Check sheet for the drawn part. Datum: minimum x, y, z corner. Units: mm. Coordinates: 2 decimals unless noted, no trailing zeros. Order: outer loops, then holes, each group sorted by start corner. A loop starts at its lowest first (then second) coordinate and runs counter-clockwise, first axis right, second up. Notation, with made-up numbers: M 28,-10 L 42,-10 A25 ccw 42,9 Z; hole C 60.25,20 d4. An arc over 180 degrees is marked long. Answer in a Markdown table with one row per item. Add a question column.
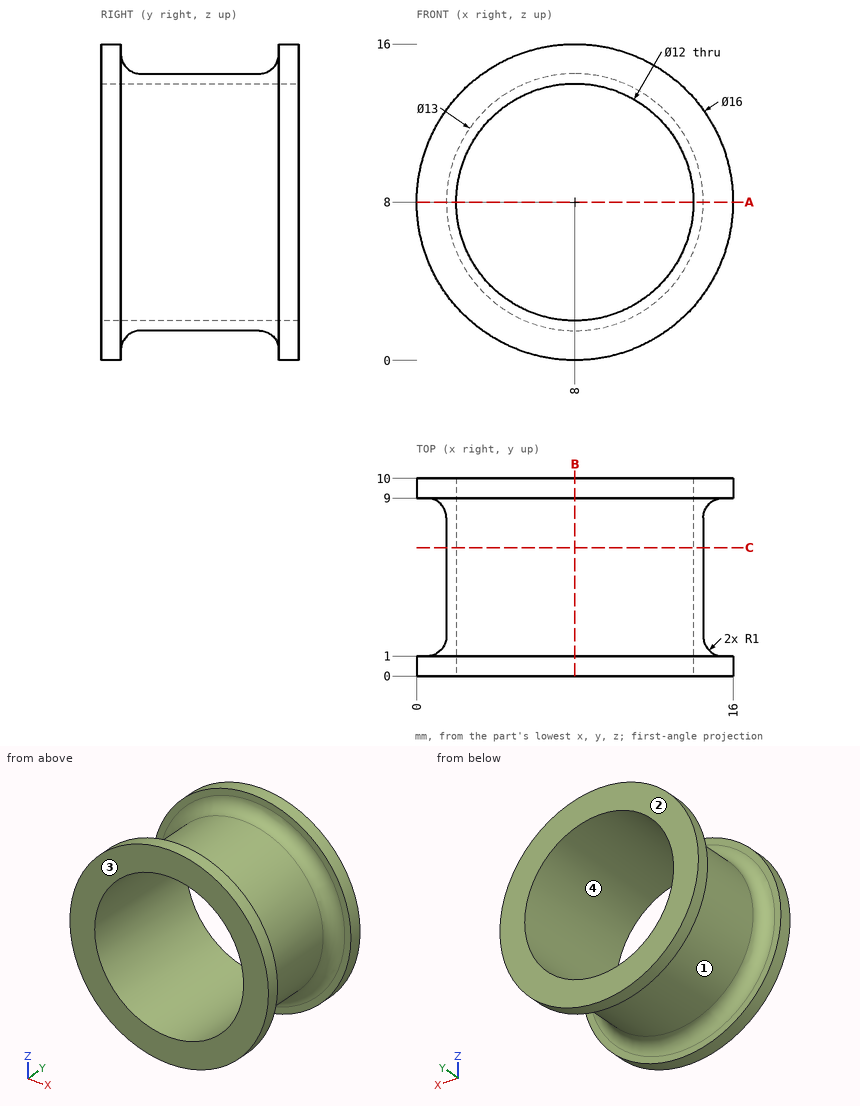
1. Section check C-C on y = 6.5. Enter the section's corners in (x, z), then the cut area to 3 significant figures.
2. Section check B-B on x = 8. Enter the section's corners in (y, z).
3. Release check for a two-part mould opening along Y. For the marked faces 1, 2, 3 and 4 record: released by +Y, released by -Y, zero draft, split by the parting line, or undercut.
4. Scan lines: line 1 (X direction, y = 2.75, z = 8); line 2 (Y direction, x = 12.75, z = 14.25); line 3 (Y direction, x = 1.75, z = 4.75). Record each from-to range of solid material in increasing order.
5. Section check A-A on z = 8. Enter the section's corners in (x, y).
6. Go/stop test with flat-tipped pins: pin 1 Ø1 at (y, z) = (2, 5) entering from +X; pin 2 Ø6 at (x, y) = (4.5, 7) entering from -Z. Record where each tip stops, or that it passes through.
Result sheet:
| question | item | result |
|---|---|---|
| 1 | outline | C 8,8 d13; hole C 8,8 d12 |
| 1 | area | 19.6 mm^2 |
| 2 | outline | M 0,0 L 1,0 L 1,0.5 A1 cw 2,1.5 L 8,1.5 A1 cw 9,0.5 L 9,0 L 10,0 L 10,2 L 0,2 Z; M 0,14 L 10,14 L 10,16 L 9,16 L 9,15.5 A1 cw 8,14.5 L 2,14.5 A1 cw 1,15.5 L 1,16 L 0,16 Z |
| 3 | face 1 | undercut |
| 3 | face 2 | released by +Y |
| 3 | face 3 | released by -Y |
| 3 | face 4 | zero draft |
| 4 | line 1 | 1.5 to 2, 14 to 14.5 |
| 4 | line 2 | 0 to 1, 9 to 10 |
| 4 | line 3 | 0 to 1.11, 8.89 to 10 |
| 5 | outline | M 0,0 L 2,0 L 2,10 L 0,10 L 0,9 L 0.5,9 A1 cw 1.5,8 L 1.5,2 A1 cw 0.5,1 L 0,1 Z; M 14,0 L 16,0 L 16,1 L 15.5,1 A1 cw 14.5,2 L 14.5,8 A1 cw 15.5,9 L 16,9 L 16,10 L 14,10 Z |
| 6 | pin 1 | x = 14.01 |
| 6 | pin 2 | z = 0.1 |
